Work out the finished part from the listing and answer in its coordinate system (mm). Face numbers are marked on the shaded views. A direction names the side the tool comes from. Round coordinates to 2 decimals unless told otherwise and drop trailing zeros. Write each loop counter-clockwise with the first axis right and the second up, starting at its lowest first coordinate (ties: lowest second). Pieces come first, ordered by that corner, then holes.
1. Determine the mould class of the marked faces 1, 2 and 3 for opening direction Y: pulls with the +Y half, pulls with the -Y half, needs draft (parallel to the pull), parting line crosses it, or undercut.
2. Flat-ended cylindrical pins translate along their axes: pin 1 Ø10 at (y, z) = (55, -79) entering from -X; pin 2 Ø1 at (x, z) = (84.5, -93.5) entering from +Y; pin 3 Ø2 at (x, y) = (160, 51) entering from +Z. Find the tip coordinate at first contact, or state that the pin passes through.
3. Straight lines are drawn through the part: probe 1 along Y at (x, z) = (159.5, -59); probe 2 along X at (y, z) = (9, 93); probe 3 along Y at (x, z) = (96, -39). For each, find the intervals that lie inside material, in ascending order.
4. A tool of negligible diameter and unlimited length cuts with its end or side. For the marked faces 4, 5 and 6, from which of +Z, -Z, +X, -X, +Y, -Y can it reach the whole face along a straight path? Write none if from no direction.
5. Find section C-C (y = 61). Write down the section's boundary in (x, z), and give its area (3 significant figures).
6. Find section A-A (x = 176.5). Write down the section's boundary in (y, z), and give its area (3 significant figures).
7. Find section B-B (z = 8.5). Write down the section's boundary in (x, y).
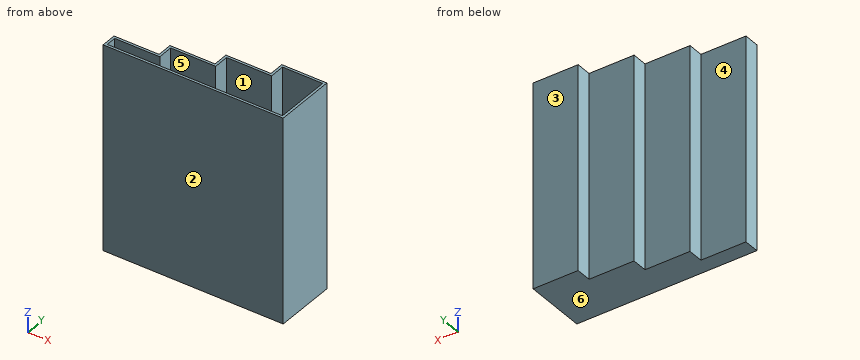
```python
from build123d import *

# Parameters (mm, degrees)
BOSS_EXTRUDE1_DEPTH = 125
SHELL1_T            = -3


with BuildPart() as part:
    # Sketch1 → Boss-Extrude1 (new, symmetric)
    with BuildSketch(Plane.XY):
        Polygon((0, 0), (0, 18.75), (55, 18.75), (55, 37.5), (110, 37.5), (110, 56.25), (165, 56.25), (165, 75), (220, 75), (220, 0), align=None)
    extrude(amount=BOSS_EXTRUDE1_DEPTH, both=True)

    # Shell1
    shell1_openings = [part.faces().sort_by_distance(p)[0] for p in [
        (137.5, 28.125, 125),
    ]]
    offset(amount=SHELL1_T, openings=shell1_openings, kind=Kind.INTERSECTION)


solid = part.part
```
Worked answers:
1. face 1: undercut
1. face 2: pulls with the -Y half
1. face 3: pulls with the +Y half
2. pin 1: stops at x = 110
2. pin 2: stops at y = 37.5
2. pin 3: stops at z = -122
3. probe 1: y = 0 to 3, 53.25 to 56.25
3. probe 2: x = 0 to 3, 217 to 220
3. probe 3: y = 0 to 3, 34.5 to 37.5
4. face 4: +Z, -Z, -X, +Y
4. face 5: +Z
4. face 6: -Z, +X, -X, +Y, -Y
5. outline: (165, -125) - (220, -125) - (220, 125) - (217, 125) - (217, -122) - (168, -122) - (168, 125) - (165, 125) - close
5. area: 1,650 mm2
6. outline: (0, -125) - (75, -125) - (75, 125) - (72, 125) - (72, -122) - (3, -122) - (3, 125) - (0, 125) - close
6. area: 1,710 mm2
7. outline: (0, 0) - (220, 0) - (220, 75) - (165, 75) - (165, 56.25) - (110, 56.25) - (110, 37.5) - (55, 37.5) - (55, 18.75) - (0, 18.75) - close; hole (3, 3) - (217, 3) - (217, 72) - (168, 72) - (168, 53.25) - (113, 53.25) - (113, 34.5) - (58, 34.5) - (58, 15.75) - (3, 15.75) - close
